Solid Edge part; units mm, degrees
sketch "Sketch1" plane through (0, 0, 0) normal (0, -1, 0) x (1, 0, 0)
  line L0 (0, 0) -> (-20, 0)
  line L1 (-20, 0) -> (-20, 12)
  line L2 (-20, 12) -> (-65, 12)
  line L3 (-65, 12) -> (-65, 0)
  line L4 (-65, 0) -> (-85, 0)
  line L5 (-85, 0) -> (-85, 95)
  line L6 (-85, 95) -> (-55, 95)
  line L7 (-55, 95) -> (-55, 60)
  line L8 (0, 35) -> (-55, 60)
  line L9 (0, 0) -> (0, 35)
extrude "ProtrusiónExtruida_1" add sketch "Sketch1" along normal blind 64
sketch "Sketch2" plane through (-85, -32, 47.5) normal (-1, 0, 0) x (0, -1, 0)
  line L0 (-20, 30.5) -> (20, 30.5)
  line L1 (20, 30.5) -> (20, -30.5)
  line L2 (-20, -30.5) -> (20, -30.5)
  line L3 (-20, 30.5) -> (-20, -30.5)
extrude "VaciadoExtruido_1" cut sketch "Sketch2" against normal blind 85
Design review of the part built by this model. Coordinates are the model's own, in mm. A direction names the side the tool comes from. Give positions to 0.01 mm unless a question says otherwise; leave off trailing zeros. Loops run counter-clockwise (first coordinate to the right, second up) from the corner with the lowest first, then second, coordinate; pieces in that order, holes last. Notation, with made-up numbers: M -7.75,-3.75 L 3.25,-3.75 A22 ccw 3.25,24.25 Z; hole C -26.5,0 d9. An arc over 180 degrees is marked long. Answer as a JSON object with one key per item and string values.
Item 1: We need section A-A (z = 18.5). State the section outline as (x, y) points.
Output values:
{"outline": "M -85,-64 L 0,-64 L 0,-52 L -85,-52 Z; M -85,-12 L 0,-12 L 0,0 L -85,0 Z"}
Item 2: Machinability: for faces 5 (the face through (0, -32, 13)), 6 (the face through (-53, -12, 41)), 7 (the face through (-65, -32, 6)), 8 (the face through (-55, -32, 82)), which of the approach directions +Z, -Z, +X, -X, +Y, -Y give a long, thin tool a straight path to every point of the face, cutting with its end or side? Answer none if there is none.
Output values:
{"face 5": "+Z, -Z, +X, +Y, -Y", "face 6": "+X, -X", "face 7": "-Z, +Y, -Y", "face 8": "+Z, +X, +Y, -Y"}
Item 3: We need section C-C (x = -77). State the section outline as (y, z) points.
Output values:
{"outline": "M -64,0 L 0,0 L 0,95 L -64,95 Z; hole M -52,17 L -12,17 L -12,78 L -52,78 Z"}
Item 4: For P1, Ø10, axis at x = -28.5, y = -47, coming from the -Z side; P2, Ø6, axis at y = -52.5, z = 45.5, coming from the +X side; P3, Ø8, axis at x = -15, y = -27, coming from the +Z side, all flat-tipped, find the tip position at first contact; note any pin that passes through.
Output values:
{"P1": "stops at z = 12", "P2": "stops at x = -16.5", "P3": "stops at z = 17"}
Item 5: Wall thickness on line 1 along Z through (x, y) = (-63, -39); line 2 along Z through (x, y) = (-71.5, -29); line 3 along Y through (x, z) = (-10, 30.5): over which ranges is each line inside the solid? List them lowest first.
Output values:
{"line 1": "z = 12 to 17, 78 to 95", "line 2": "z = 0 to 17, 78 to 95", "line 3": "y = -64 to -52, -12 to 0"}
Item 6: Mouldability with a two-part tool opening along Z and no side actions: class faces 1 (the face through (-51, 0, 36)), 2 (the face through (-27.115, -5.916, 47.325)), 3 (the face through (-43, -32, 17)), 4 (the face through (-42, -32, 12)) as pulls with the +Z half, pulls with the -Z half, needs draft (parallel to the pull), parting line crosses it, or undercut.
Output values:
{"face 1": "needs draft", "face 2": "pulls with the +Z half", "face 3": "undercut", "face 4": "pulls with the -Z half"}
Item 7: We need section D-D (y = -58.5). State the section outline as (x, z) points.
Output values:
{"outline": "M -85,0 L -65,0 L -65,12 L -20,12 L -20,0 L 0,0 L 0,35 L -55,60 L -55,95 L -85,95 Z"}
Item 8: We need section B-B (y = -31). State the section outline as (x, z) points, and give its area (4 significant figures).
Output values:
{"outline": "M -85,0 L -65,0 L -65,12 L -20,12 L -20,0 L 0,0 L 0,17 L -85,17 Z; M -85,78 L -55,78 L -55,95 L -85,95 Z", "area": "1,415 mm2"}
